Part model, mm, in its own coordinate system. A direction names the side the tool comes from. Round coordinates to 2 decimals unless told otherwise and drop trailing zeros. Order: outer loops, then holes, each group sorted by start corner. A loop starts at its lowest first (then second) coordinate and runs counter-clockwise, first axis right, second up. Notation, with made-up numbers: (-33, 66.25) - (-9, 66.25) arc R18 cw to (-9, 94.25) - close; hole circle Ø11 at (10, -12). An arc over 180 degrees is marked (long way). Return JSON: item names as keys, results as strings. Group by question number.
Item 1: Two-plate mould, pull along Z, no slides. Class faces 1 (the face through (-15, 2, 33)), 2 (the face through (-0.314, 1.565, -21.084)), 3 (the face through (5, 2, -37.5)): released by +Z, released by -Z, zero draft, split by the parting line, or undercut.
Item 2: Saw through at B-B on z = -22.5. List the corners of the cut face in (x, y) (3 decimals), and give its area (3 significant figures).
Item 3: Saw through at C-C on x = 14. List the corners of the cut face in (y, z) (3 decimals), and give its area (3 significant figures).
Item 4: Tool access for faces 4 (the face through (-12.1, 1.6, -24.6)), 5 (the face through (21.339, 1.565, -31.945)), 6 (the face through (22.9, 1.6, 25.4)): list every direction of +Z, -Z, +X, -X, +Y, -Y with a clear straight run to the whole face (end or side of a thin tool).
Item 5: Saw through at D-D on y = 1.2. State how many separate pieces and enclosed holes the cut face has, and give its area (3 significant figures).
Item 6: Saw through at A-A on x = -10. List the corners of the cut face in (y, z) (3 decimals), and give its area (3 significant figures).
Item 7: Probe probe 1 along Z at (x, y) = (20, 2.25); probe 2 along Z at (x, y) = (0, 1.3); probe 3 along X at (y, z) = (1.9, -32.5). List the from-to ranges inside material, lowest first.
```python
from build123d import *

# Parameters (mm, degrees)
SKETCH1_R           = 1.45
BOSS_EXTRUDE1_DEPTH = 3.175
CHAMFER1_SIZE       = 4.2
CHAMFER2_SIZE       = 3


with BuildPart() as part:
    # Sketch1 → Boss-Extrude1 (new body)
    with BuildSketch(Plane(origin=(0, 0, 0), x_dir=(1, 0, 0), z_dir=(0, 1, 0))):
        Polygon((5, 23.3), (25, 23.3), (25, 37.5), (-15, 37.5), (-15, 27.5), (-9.2, 21.7), (-9.2, 0), (5, 0), align=None)
        with Locations((0, 22.5)):
            Circle(SKETCH1_R, mode=Mode.SUBTRACT)
        with Locations((-10, 32.5)):
            Circle(SKETCH1_R, mode=Mode.SUBTRACT)
        with Locations((20, 32.5)):
            Circle(SKETCH1_R, mode=Mode.SUBTRACT)
        with Locations((0, 32.5)):
            Circle(SKETCH1_R, mode=Mode.SUBTRACT)
        with Locations((10, 32.5)):
            Circle(SKETCH1_R, mode=Mode.SUBTRACT)
    boss_extrude1 = extrude(amount=BOSS_EXTRUDE1_DEPTH)

    # Mirror1: Boss-Extrude1 across plane
    add(boss_extrude1.mirror(Plane(origin=(5, 3.175, 0), x_dir=(1, 0, 0), z_dir=(0, 0, -1))))

    # Chamfer1
    chamfer1_edges = [part.edges().sort_by_distance(p)[0] for p in [
        (25, 1.5875, -23.3),
        (25, 1.5875, 23.3),
    ]]
    chamfer(chamfer1_edges, length=CHAMFER1_SIZE)

    # Chamfer2
    chamfer2_edges = [part.edges().sort_by_distance(p)[0] for p in [
        (5, 1.5875, -23.3),
        (5, 1.5875, 23.3),
    ]]
    chamfer(chamfer2_edges, length=CHAMFER2_SIZE)


solid = part.part
```
Filled in:
{
 "1": {"face 1": "zero draft", "face 2": "undercut", "face 3": "released by -Z"},
 "2": {"outline": "(-10, 0) - (-1.45, 0) - (-1.45, 3.175) - (-10, 3.175) - close; (1.45, 0) - (7.2, 0) - (7.2, 3.175) - (1.45, 3.175) - close", "area": "45.4 mm^2"},
 "3": {"outline": "(0, -37.5) - (3.175, -37.5) - (3.175, -23.3) - (0, -23.3) - close; (0, 23.3) - (3.175, 23.3) - (3.175, 37.5) - (0, 37.5) - close", "area": "90.2 mm^2"},
 "4": {"face 4": "-X, +Y, -Y", "face 5": "+Y, -Y", "face 6": "+X, +Y, -Y"},
 "5": {"separate pieces": "1", "enclosed holes": "10", "area": "1,710 mm^2"},
 "6": {"outline": "(0, -37.5) - (3.175, -37.5) - (3.175, -33.95) - (0, -33.95) - close; (0, -31.05) - (3.175, -31.05) - (3.175, -22.5) - (0, -22.5) - close; (0, 22.5) - (3.175, 22.5) - (3.175, 31.05) - (0, 31.05) - close; (0, 33.95) - (3.175, 33.95) - (3.175, 37.5) - (0, 37.5) - close", "area": "76.8 mm^2"},
 "7": {"probe 1": "z = -37.5 to -33.95, -31.05 to -23.3, 23.3 to 31.05, 33.95 to 37.5", "probe 2": "z = -37.5 to -33.95, -31.05 to -23.95, -21.05 to 21.05, 23.95 to 31.05, 33.95 to 37.5", "probe 3": "x = -15 to -11.45, -8.55 to -1.45, 1.45 to 8.55, 11.45 to 18.55, 21.45 to 25"}
}
